Could you check a few things on this drawing? It's one solid part, dimensions in mm from its lowest x, y, z. A direction names the side the tool comes from. Coordinates: 2 decimals unless noted, no trailing zeros. Write each loop counter-clockwise with the first axis right and the second up, starting at its lowest first coordinate (ties: lowest second). Pieces come first, ordered by that corner, then holes.
Item 1: I'm going to push flat-ended pins straight in: P1, Ø1.5, axis at x = 8, z = 12.5, coming from the -Y side; P2, Ø0.6, axis at y = 3, z = 3.5, coming from the -X side; P3, Ø2, axis at y = 2.5, z = 12.5, coming from the +X side. Where does each tip first touch, or does it pass through?
Item 2: I want a section at D-D (z = 2). Please give me the cut outline in (x, y), and give its area (3 significant figures).
Item 3: I want a section at C-C (y = 1.25). Please give me the cut outline in (x, z), and give its area (3 significant figures).
Item 4: If we mould it in two halves opening along Z, with no side actions, what happens to the marked faces 5, 6 and 7? For each: pulls with the +Z half, pulls with the -Z half, needs draft (parallel to the pull), parting line crosses it, or undercut.
Item 5: For the marked faces 1, 2, 3 and 4, which set-ups out of +Z, -Z, +X, -X, +Y, -Y let a thin tool reach every point of the face, with its end or its side?
Item 6: Please list where these lines run through material, in increasing order: line 1 (X direction, y = 2.25, z = 8); line 2 (X direction, y = 1.05, z = 8); line 3 (Z direction, x = 15.25, y = 2.7).
Item 7: I want a section at A-A (x = 8). Please give me the cut outline in (y, z), and give its area (3 significant figures).
Item 8: I want a section at B-B (z = 8). Please give me the cut outline in (x, y).
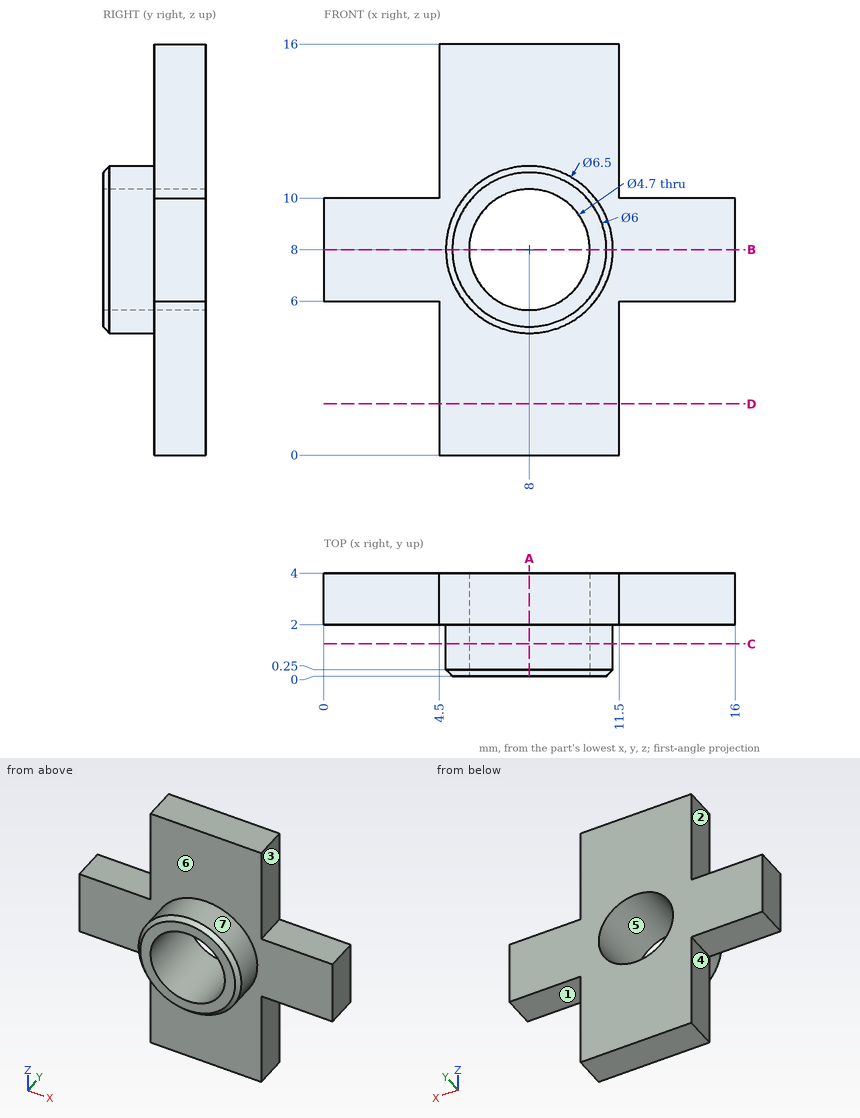
Answer:
1. P1: stops at y = 2
1. P2: stops at x = 4.5
1. P3: stops at x = 11.5
2. outline: (4.5, 2) - (11.5, 2) - (11.5, 4) - (4.5, 4) - close
2. area: 14.0 mm2
3. outline: circle Ø6.5 at (8, 8); hole circle Ø4.7 at (8, 8)
3. area: 15.8 mm2
4. face 5: undercut
4. face 6: needs draft
4. face 7: parting line crosses it
5. face 1: -Z, +X, +Y, -Y
5. face 2: +Z, -X, +Y, -Y
5. face 3: +Z, +X, +Y, -Y
5. face 4: -Z, -X, +Y, -Y
6. line 1: x = 0 to 5.65, 10.35 to 16
6. line 2: x = 4.75 to 5.65, 10.35 to 11.25
6. line 3: z = 6 to 10
7. outline: (0, 5) - (0.25, 4.75) - (2, 4.75) - (2, 0) - (4, 0) - (4, 5.65) - (0, 5.65) - close; (0, 10.35) - (4, 10.35) - (4, 16) - (2, 16) - (2, 11.25) - (0.25, 11.25) - (0, 11) - close
7. area: 26.1 mm2
8. outline: (0, 2) - (4.75, 2) - (4.75, 0.25) - (5, 0) - (5.65, 0) - (5.65, 4) - (0, 4) - close; (10.35, 0) - (11, 0) - (11.25, 0.25) - (11.25, 2) - (16, 2) - (16, 4) - (10.35, 4) - close
